from build123d import *

# Parameters (mm, degrees)
F0_W     = 61
F0_H     = 40
F0_R     = 1.6
F0_R_2   = 2.6
F1_DEPTH = 8
F2_R     = 5
F2_R_2   = 2.6
F3_DEPTH = 3
F4_R     = 1.6
F5_DEPTH = 4
F6_R     = 5


with BuildPart() as f1:
    # F0 (on Top) → F1 (new body)
    with BuildSketch(Plane.XY):
        Rectangle(F0_W, F0_H)
        with Locations((-9.9, -15.4)):
            Circle(F0_R, mode=Mode.SUBTRACT)
        with Locations((-22.5, -10)):
            Circle(F0_R_2, mode=Mode.SUBTRACT)
        with Locations((9.9, -15.4)):
            Circle(F0_R, mode=Mode.SUBTRACT)
        with Locations((22.5, -10)):
            Circle(F0_R_2, mode=Mode.SUBTRACT)
        with Locations((-22.5, 10)):
            Circle(F0_R_2, mode=Mode.SUBTRACT)
        with Locations((-9.9, 15.4)):
            Circle(F0_R, mode=Mode.SUBTRACT)
        with Locations((9.9, 15.4)):
            Circle(F0_R, mode=Mode.SUBTRACT)
        with Locations((22.5, 10)):
            Circle(F0_R_2, mode=Mode.SUBTRACT)
    extrude(amount=F1_DEPTH)

    # F2 (on face) → F3 (cut)
    with BuildSketch(Plane.XY.offset(8)):
        with Locations((-22.5, 10)):
            Circle(F2_R)
        with Locations((-22.5, 10)):
            Circle(F2_R_2, mode=Mode.SUBTRACT)
        with Locations((22.5, 10)):
            Circle(F2_R)
        with Locations((22.5, 10)):
            Circle(F2_R_2, mode=Mode.SUBTRACT)
        with Locations((22.5, -10)):
            Circle(F2_R)
        with Locations((22.5, -10)):
            Circle(F2_R_2, mode=Mode.SUBTRACT)
        with Locations((-22.5, -10)):
            Circle(F2_R)
        with Locations((-22.5, -10)):
            Circle(F2_R_2, mode=Mode.SUBTRACT)
    extrude(amount=-F3_DEPTH, mode=Mode.SUBTRACT)

    # F4 (on face) → F5 (cut)
    with BuildSketch(Plane(origin=(0, 0, 0), x_dir=(1, 0, 0), z_dir=(0, 0, -1))):
        Polygon((-8.167949, 18.4), (-11.632051, 18.4), (-13.364102, 15.4), (-11.632051, 12.4), (-8.167949, 12.4), (-6.435898, 15.4), align=None)
        with Locations((-9.9, 15.4)):
            Circle(F4_R, mode=Mode.SUBTRACT)
        Polygon((11.632051, 18.4), (8.167949, 18.4), (6.435898, 15.4), (8.167949, 12.4), (11.632051, 12.4), (13.364102, 15.4), align=None)
        with Locations((9.9, 15.4)):
            Circle(F4_R, mode=Mode.SUBTRACT)
        Polygon((-8.167949, -12.4), (-11.632051, -12.4), (-13.364102, -15.4), (-11.632051, -18.4), (-8.167949, -18.4), (-6.435898, -15.4), align=None)
        with Locations((-9.9, -15.4)):
            Circle(F4_R, mode=Mode.SUBTRACT)
        Polygon((8.167949, -18.4), (11.632051, -18.4), (13.364102, -15.4), (11.632051, -12.4), (8.167949, -12.4), (6.435898, -15.4), align=None)
        with Locations((9.9, -15.4)):
            Circle(F4_R, mode=Mode.SUBTRACT)
    extrude(amount=-F5_DEPTH, mode=Mode.SUBTRACT)

    # F6
    f6_edges = [f1.edges().sort_by_distance(p)[0] for p in [
        (-30.5, 20, 4),
        (-30.5, -20, 4),
        (30.5, -20, 4),
        (30.5, 20, 4),
    ]]
    fillet(f6_edges, radius=F6_R)


solid = f1.part
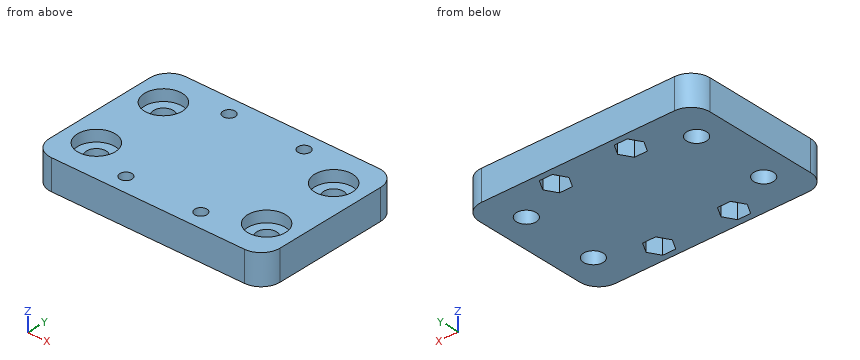
CAD build for the part. Positions are in the model's coordinates, mm. Give positions to 0.01 mm unless a question says otherwise; leave off trailing zeros. Write each loop counter-clockwise with the first axis right and the second up, starting at its lowest first coordinate (ties: lowest second). Pieces come first, ordered by that corner, then holes. Notation, with made-up numbers: (58.5, 23.25) -> (87.5, 23.25) arc R19 cw to (87.5, 29.25) -> close; hole circle Ø2 at (53, 57). An arc over 180 degrees is marked (long way). Return JSON: item names as keys, results as strings.
Item 1: Band-saw the part on A-A (x = 9.9). List the corners of the cut face in (y, z), then the cut area to 3 significant figures.
Answer below:
{"outline": "(-20, 0) -> (-18.4, 0) -> (-18.4, 4) -> (-17, 4) -> (-17, 8) -> (-20, 8) -> close; (-13.8, 4) -> (-12.4, 4) -> (-12.4, 0) -> (12.4, 0) -> (12.4, 4) -> (13.8, 4) -> (13.8, 8) -> (-13.8, 8) -> close; (17, 4) -> (18.4, 4) -> (18.4, 0) -> (20, 0) -> (20, 8) -> (17, 8) -> close", "area": "246 mm2"}
Item 2: Band-saw the part on B-B (z = 6.75). Give the number of separate pieces and of enclosed holes in the cut face, then the cut area to 3 significant figures.
Answer below:
{"separate pieces": "1", "enclosed holes": "8", "area": "2,070 mm2"}
Item 3: Band-saw the part on C-C (y = 8.5). List the corners of the cut face in (x, z), then the cut area to 3 significant figures.
Answer below:
{"outline": "(-30.5, 0) -> (-24.62, 0) -> (-24.62, 5) -> (-27.27, 5) -> (-27.27, 8) -> (-30.5, 8) -> close; (-20.38, 0) -> (20.38, 0) -> (20.38, 5) -> (17.73, 5) -> (17.73, 8) -> (-17.73, 8) -> (-17.73, 5) -> (-20.38, 5) -> close; (24.62, 0) -> (30.5, 0) -> (30.5, 8) -> (27.27, 8) -> (27.27, 5) -> (24.62, 5) -> close", "area": "388 mm2"}
Item 4: Drop flat-ended pins along their axis: pin 1 (1.8 mm diameter, centred on x = 9, y = 16, fed in from -Z); pin 2 (8.5 mm diameter, centred on x = 22.5, y = -10, fed in from +Z). Give the stop position or say it passes through.
Answer below:
{"pin 1": "stops at z = 4", "pin 2": "stops at z = 5"}
Item 5: Drill centre lines: probe 1 along Y at (x, z) = (22.5, 2.05); probe 2 along Y at (x, z) = (11, 1.25); probe 3 along X at (y, z) = (9.5, 1). Where is each one in solid material? Low to high.
Answer below:
{"probe 1": "y = -20 to -12.6, -7.4 to 7.4, 12.6 to 20", "probe 2": "y = -20 to -18.4, -12.4 to 12.4, 18.4 to 20", "probe 3": "x = -30.5 to -25.05, -19.95 to 19.95, 25.05 to 30.5"}
